Geometry: final body of the model. Coordinates: model frame, mm. A direction names the side the tool comes from. Round coordinates to 2 decimals unless told otherwise and drop trailing zeros. Loops run counter-clockwise (first coordinate to the right, second up) from the corner with the lowest first, then second, coordinate; pieces in that order, holes last. Notation, with made-up numbers: (17.25, 40.25) - (34.25, 40.25) arc R31 ccw to (34.25, 70.25) - close; hole circle Ø1 at (-27.75, 6). An arc over 180 degrees is marked (long way). Write item = value, one per line. Start each with the question number.
Item 1: Access query for faces 5 (the flat face through (0, -75.157, 11)), 6 (the flat face through (-10, -95.074, 11)), 7 (the flat face through (1, 0, 0)), 8 (the flat face through (-9.023, 85, 11)), 9 (the flat face through (1, -69.853, 19)). Directions: +Z, -Z, +X, -X, +Y, -Y. A direction counts if a zero-diameter tool reaches every point of the face in a straight line with its end or side. Return the directions, or none.
Item 2: Line query: line 1 (X direction, y = -80.5, z = 15); line 2 (Y direction, x = -10.5, z = 18); line 3 (Z direction, x = 4.5, y = 8). Output: solid intervals per line, ascending. Write a range as from..to.
Item 3: Section A-A (z = 18). Return loops of the section in (x, y), plus the area to 3 significant figures.
Item 4: Draft query along Y for faces 1 (the flat face through (7.3, -82.3, 25)), 2 (the flat face through (1, 61.371, 19)), 3 (the flat face through (1, -3, 15)), 4 (the flat face through (-12, 92.927, 11)). Return one class per face: pulls with the +Y half, pulls with the -Y half, needs draft (parallel to the pull), parting line crosses it, or undercut.
Item 5: First-contact query: pin 1 (8 mm diameter, centred on x = -8, y = -6.5, fed in from +Z); pin 2 (3 mm diameter, centred on x = -5.5, z = 14.5, fed in from +Y); pin 3 (4 mm diameter, centred on x = -1, z = 18, fed in from +Y); pin 4 (1 mm diameter, centred on y = 26.5, z = 16.5, fed in from -X). Flat tips, straight axial feed; report the tip coordinate or a pass-through.
Item 6: Section C-C (y = -46). Return loops of the section in (x, z).
Item 7: Section B-B (z = 9). Return loops of the section in (x, y), plus the area to 3 significant figures.
from build123d import *

# Parameters (mm, degrees)
F1_DEPTH = 25
F0_W     = 6.0739132134
F0_H     = 16.4999708235
F0_W_2   = 32.4678264267
F0_H_2   = 131.2236316204
F2_DEPTH = 15
F3_R     = 2


with BuildPart() as f1:
    # F0 (on Top) → F1 (new body)
    with BuildSketch(Plane.XY):
        Polygon((17.3710967268, -69.8527075052), (-15.0967296999, -69.8527075052), (-15.0967296999, -95.0735285878), (-3.9494665107, -95.0735285878), (-3.9494665107, -75.1573219895), (5.0167334893, -75.1573219895), (5.0167334893, -95.0735285878), (17.3710967268, -95.0735285878), align=None)
    extrude(amount=F1_DEPTH)



with BuildPart() as f1b:
    # F0 (on Top) → F1, piece 2 (new body)
    with BuildSketch(Plane.XY):
        with BuildLine():
            Line((-9.0228164865, 76.4271907806), (-15.0967296999, 76.4271907806))
            Line((-15.0967296999, 76.4271907806), (-15.0967296999, 61.3709241152))
            Line((-15.0967296999, 61.3709241152), (17.3710967268, 61.3709241152))
            Line((17.3710967268, 61.3709241152), (17.3710967268, 76.4271907806))
            Line((17.3710967268, 76.4271907806), (11.2971835135, 76.4271907806))
            ThreePointArc((11.2971835135, 76.4271907806), (1.1371835135, 66.2671907806), (-9.0228164865, 76.4271907806))
        make_face()
        with Locations((14.3341401202, 84.6771761924)):
            Rectangle(F0_W, F0_H)
        with Locations((-12.0597730932, 84.6771761924)):
            Rectangle(F0_W, F0_H)
    extrude(amount=F1_DEPTH)


with BuildPart() as f1_1:
    add(f1.part)

    add(f1b.part)  # F2 merges F1b
    # F0 (on Top) → F2 (join)
    with BuildSketch(Plane.XY):
        with Locations((1.1371835135, -4.240891695)):
            Rectangle(F0_W_2, F0_H_2)
    extrude(amount=F2_DEPTH)

    # F3
    f3_edges = [f1_1.edges().sort_by_distance(p)[0] for p in [
        (1.137184, 61.370924, 25),
        (17.371097, 77.149043, 25),
        (14.33414, 92.927162, 25),
        (11.297184, 84.677176, 25),
        (1.137184, 66.267191, 25),
        (-9.022816, 84.677176, 25),
        (-12.059773, 92.927162, 25),
        (-15.09673, 77.149043, 25),
        (17.371097, -82.463118, 25),
        (1.137184, -69.852708, 25),
        (-15.09673, -82.463118, 25),
        (-9.523098, -95.073529, 25),
        (-3.949467, -85.115425, 25),
        (0.533633, -75.157322, 25),
        (5.016733, -85.115425, 25),
        (11.193915, -95.073529, 25),
    ]]
    fillet(f3_edges, radius=F3_R)


solid = f1_1.part
Taken from the geometry:
q1.face_5 = +Z, -Z, -Y
q1.face_6 = +Z, -Z, +X, -X, -Y
q1.face_7 = -Z, +X, -X, +Y, -Y
q1.face_8 = +Z, -Z, +Y
q1.face_9 = +Z, +X, -X
q2.line_1 = -15.1..-3.95, 5.02..17.37
q2.line_2 = -95.07..-69.85, 61.37..92.93
q2.line_3 = 0..15
q3.outline = (-15.1, -95.07) - (-3.95, -95.07) - (-3.95, -75.16) - (5.02, -75.16) - (5.02, -95.07) - (17.37, -95.07) - (17.37, -69.85) - (-15.1, -69.85) - close; (-15.1, 61.37) - (17.37, 61.37) - (17.37, 92.93) - (11.3, 92.93) - (11.3, 76.43) arc R10.16 cw to (-9.02, 76.43) - (-9.02, 92.93) - (-15.1, 92.93) - close
q3.area = 1,170 mm^2
q4.face_1 = needs draft
q4.face_2 = undercut
q4.face_3 = undercut
q4.face_4 = pulls with the +Y half
q5.pin_1 = 15
q5.pin_2 = 70.34
q5.pin_3 = 67.15
q5.pin_4 = through
q6.outline = (-15.1, 0) - (17.37, 0) - (17.37, 15) - (-15.1, 15) - close
q7.outline = (-15.1, -95.07) - (-3.95, -95.07) - (-3.95, -75.16) - (5.02, -75.16) - (5.02, -95.07) - (17.37, -95.07) - (17.37, 92.93) - (11.3, 92.93) - (11.3, 76.43) arc R10.16 cw to (-9.02, 76.43) - (-9.02, 92.93) - (-15.1, 92.93) - close
q7.area = 5,430 mm^2
